```python
from build123d import *

# Parameters (mm, degrees)
BOSS_EXTRUDE1_DEPTH = 9.4
SKETCH2_R           = 2.1
CUT_EXTRUDE1_DEPTH  = 9.4
FILLET1_R           = 4


with BuildPart() as part:
    # Sketch1 → Boss-Extrude1 (new body)
    with BuildSketch(Plane.XY):
        with BuildLine():
            Line((0, -1.55), (-8.4, -1.55))
            Line((-8.4, -1.55), (-8.4, -2.85))
            Line((-8.4, -2.85), (0, -2.85))
            ThreePointArc((0, -2.85), (2.132811003, 1.89040134), (-2.829381598, 0.342198439))
            ThreePointArc((-2.829381598, 0.342198439), (-2.911748288, 0.185127161), (-3.077572967, 0.122215846))
            Line((-3.077572967, 0.122215846), (-8.4, 0.122215846))
            Line((-8.4, 0.122215846), (-8.4, -1.177784154))
            Line((-8.4, -1.177784154), (-1.302793355, -1.177784154))
            ThreePointArc((-1.302793355, -1.177784154), (-1.189997637, -1.106655539), (-1.20556997, -0.974218173))
            ThreePointArc((-1.20556997, -0.974218173), (0.668005177, 1.398666895), (0, -1.55))
        make_face()
    extrude(amount=BOSS_EXTRUDE1_DEPTH)

    # Sketch2 → Cut-Extrude1 (cut)
    with BuildSketch(Plane(origin=(0, 0.122215846, 0), x_dir=(1, 0, 0), z_dir=(0, 1, 0))):
        with Locations((-5.738786483, -4.7)):
            Circle(SKETCH2_R)
    extrude(amount=-CUT_EXTRUDE1_DEPTH, mode=Mode.SUBTRACT)

    # Fillet1
    fillet1_edges = [part.edges().sort_by_distance(p)[0] for p in [
        (-8.4, -0.527784154, 0),
        (-8.4, -2.2, 0),
        (-8.4, -2.2, 9.4),
        (-8.4, -0.527784154, 9.4),
    ]]
    fillet(fillet1_edges, radius=FILLET1_R)


solid = part.part
```
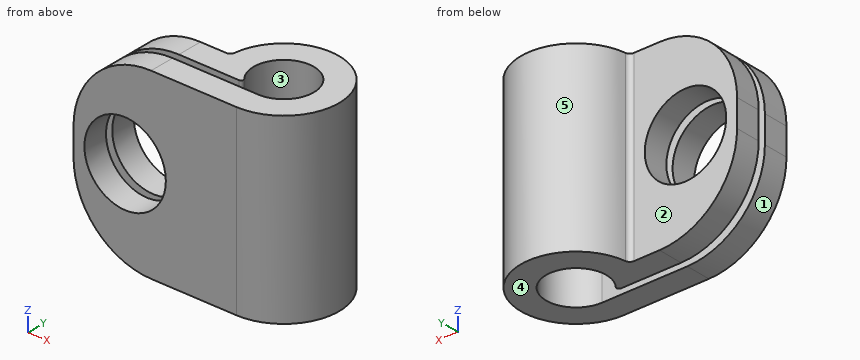
Here's how the part is built. I have some questions about the finished solid (model axes, mm). Face numbers are marked on the shaded views. A direction names the side the tool comes from. Round coordinates to 2 decimals unless told otherwise and drop trailing zeros. Order: outer loops, then holes, each group sorted by start corner. A loop starts at its lowest first (then second) coordinate and runs counter-clockwise, first axis right, second up. Notation, with made-up numbers: M 73,71 L 107,71 A20 ccw 107,77 Z; hole C -27.75,59 d1. An arc over 180 degrees is marked long. Use CSV: the item, a comma, the result in double quotes.
1) On a 3-axis mill with a long thin cutter (end or side, diameter ignored), from which of +Z, -Z, +X, -X, +Y, -Y can I reach the whole of each face in a straight line? I mean the marked faces 1 and 2. Say none if no direction works.
Taken from the geometry:
face 1,"-Z, -X, +Y, -Y"
face 2,"+Z, -Z, -X, +Y"
2) I want a section at C-C (x = -0.25). List the corners of the cut face in (y, z) for me.
Taken from the geometry:
outline,"M -2.85,0 L -1.55,0 L -1.55,9.4 L -2.85,9.4 Z; M 1.53,0 L 2.84,0 L 2.84,9.4 L 1.53,9.4 Z"
3) I want a section at D-D (y = -1.9). List the corners of the cut face in (x, z) for me, then the cut area to 3 significant figures.
Taken from the geometry:
outline,"M -8.4,4 A4 ccw -4.4,0 L 2.12,0 L 2.12,9.4 L -4.4,9.4 A4 ccw -8.4,5.4 Z; hole C -5.74,4.7 d4.2"
area,"78.2 mm^2"
4) If we mould it in two halves opening along Y, with no side actions, what happens to the marked faces 3, 4 and 5? For each: pulls with the +Y half, pulls with the -Y half, needs draft (parallel to the pull), parting line crosses it, or undercut.
Taken from the geometry:
face 3,"undercut"
face 4,"needs draft"
face 5,"parting line crosses it"
5) I'm going to push flat-ended pins straight in: P1, Ø5, axis at x = -5.74, z = 4.7, coming from the +Y side; P2, Ø1, axis at y = -1.5, z = 6, coming from the -X side; P3, Ø3, axis at y = 2, z = 5.5, coming from the +X side. Where does each tip first touch, or does it pass through?
Taken from the geometry:
P1,"y = 0.12"
P2,"x = -8.4"
P3,"x = 2.81"
6) I need wall thicknesses on line 1 along Y through (x, z) = (-3.75, 7.5); line 2 along X through (y, z) = (0, 4); line 3 along X through (y, z) = (0, 3.5). Which ranges of each line are inside material? Lowest first, please. Write a range as [from, to].
Taken from the geometry:
line 1,"[-2.85, -1.55], [-1.18, 0.12]"
line 2,"[-8.4, -7.72], [-3.76, -1.55], [1.55, 2.85]"
line 3,"[-8.37, -7.46], [-4.02, -1.55], [1.55, 2.85]"
7) I want a section at A-A (y = -0.75). List the corners of the cut face in (x, z) for me.
Taken from the geometry:
outline,"M -8.4,4 A4 ccw -4.4,0 L -1.36,0 L -1.36,9.4 L -4.4,9.4 A4 ccw -8.4,5.4 Z; M 1.36,0 L 2.75,0 L 2.75,9.4 L 1.36,9.4 Z; hole C -5.74,4.7 d4.2"
8) I want a section at B-B (z = 3.25). List the corners of the cut face in (x, y) for me (3 decimals), then the cut area to 3 significant figures.
Taken from the geometry:
outline,"M -8.329,-2.85 L -7.258,-2.85 L -7.258,-1.55 L -8.329,-1.55 Z; M -8.329,-1.178 L -7.258,-1.178 L -7.258,0.122 L -8.329,0.122 Z; M -4.22,-2.85 L 0,-2.85 A2.85 ccw long -2.829,0.342 A0.25 cw -3.078,0.122 L -4.22,0.122 L -4.22,-1.178 L -1.303,-1.178 A0.125 ccw -1.206,-0.974 A1.55 cw long 0,-1.55 L -4.22,-1.55 Z"
area,"25.2 mm^2"
